Build history of the part. All positions in model axes, mm. A direction names the side the tool comes from. Give positions to 0.01 mm unless a question says otherwise; leave off trailing zeros. Order: outer loops, then holes, each group sorted by start corner. A loop starts at its lowest first (then second) coordinate and runs counter-clockwise, first axis right, second up. Notation, with made-up numbers: (58.25, 11.25) - (111.25, 11.25) arc R17 cw to (111.25, 30.25) - close; hole circle Ø9 at (74, 55). An arc over 180 degrees is marked (long way). Write each question's results on one line, items separated by ' | '. Start each with the question number.
1) Drill centre lines: line 1 along Y through (x, z) = (-4.5, 14); line 2 along Z through (x, y) = (0, 87.5); line 3 along X through (y, z) = (70.5, 50). Where is each one in solid material? Low to high. Write a range as from..to.
2) Drop flat-ended pins along their axis: pin 1 Ø2 at (x, z) = (-12.5, -1) entering from +Y; pin 2 Ø15.5 at (x, z) = (-1.5, 39) entering from +Y; pin 3 Ø3 at (x, y) = (15, 98) entering from +Z; pin 4 Ø6 at (x, z) = (3, -36.5) entering from +Y. Give the stop position or say it passes through.
3) Cut at C-C on y = 81. List the corners of the cut face in (x, z), plus the area to 3 significant figures.
4) Tool access for faces 1 (the face through (13, 100, 44)), 2 (the face through (-4, 5.68, 4)), 3 (the face through (-0.66, 21.367, 14.985)): list every direction of +Z, -Z, +X, -X, +Y, -Y with a clear straight run to the whole face (end or side of a thin tool).
5) Two-plate mould, pull along Y, no slides. Class faces 4 (the face through (0.252, 13.804, -36.289)), 5 (the face through (0.252, 69.587, -44.867)), 6 (the face through (0, 63, 19)), 7 (the face through (-13, 100, 44)): +Y half, -Y half, draft (parallel to the pull), parting line (faces both ways), or undercut.
6) Cut at D-D on x = -2. State how many separate pieces and enclosed holes the cut face has, plus the area to 3 significant figures.
7) Cut at A-A on y = 41. List the corners of the cut face in (x, z).
8) Cut at B-B on z = 47. List the corners of the cut face in (x, y).
from build123d import *

# Parameters (mm, degrees)
SKETCH3_W                               = 40
SKETCH3_H                               = 12
BOSS_EXTRUDE1_DEPTH                     = 12
SKETCH5_R                               = 20
BOSS_EXTRUDE2_DEPTH                     = 20
BOSS_EXTRUDE2_DIRECTION_2_REACH         = 94.331
SKETCH7_R                               = 11.5
BOSS_EXTRUDE4_DEPTH                     = 31
SKETCH8_R                               = 15
BOSS_EXTRUDE5_DEPTH                     = 19
SKETCH9_R                               = 9
CUT_EXTRUDE1_DEPTH                      = 32
BOSS_EXTRUDE6_START                     = 10
BOSS_EXTRUDE6_DEPTH                     = 10
CBORE_FOR_M8_HEX_HEAD_BOLT1_D           = 10
CBORE_FOR_M8_HEX_HEAD_BOLT1_DEPTH       = 43
CBORE_FOR_M8_HEX_HEAD_BOLT1_CBORE_D     = 18.01
CBORE_FOR_M8_HEX_HEAD_BOLT1_CBORE_DEPTH = 5.68
CBORE_FOR_M8_HEX_HEAD_BOLT1_TIP         = 3.004303095
FILLET2_R                               = 18
FILLET3_R                               = 2
FILLET4_R                               = 6
FILLET5_R                               = 2


with BuildPart() as part:
    # Sweep1: sweep along a path in Sketch2
    with BuildLine(Plane(origin=(0, 0, 0), x_dir=(0, 0, -1), z_dir=(1, 0, 0))) as sweep1_path:
        Line((0, 0), (50, 0))
        Line((50, 0), (50, 75))
        Line((50, 75), (-50, 75))
    # Sketch3 → Sweep1 (sweep)
    with BuildSketch(Plane.XY):
        with Locations((0, 6)):
            Rectangle(SKETCH3_W, SKETCH3_H)
    sweep(path=sweep1_path.line, transition=Transition.RIGHT)

    # Sketch4 → Boss-Extrude1 (add)
    with BuildSketch(Plane(origin=(0, 12, 0), x_dir=(1, 0, 0), z_dir=(0, 1, 0))):
        with BuildLine():
            Line((-20, 0), (20, 0))
            ThreePointArc((20, 0), (0, -20), (-20, 0))
        make_face()
    extrude(amount=-BOSS_EXTRUDE1_DEPTH)

    # Sketch5 → Boss-Extrude2 (add)
    with BuildSketch(Plane(origin=(0, 75, 0), x_dir=(1, 0, 0), z_dir=(0, 1, 0))):
        with Locations(Location((0, -50, 0), (0, 0, 270))):
            Circle(SKETCH5_R)
    extrude(amount=BOSS_EXTRUDE2_DEPTH)

    # Boss-Extrude2 direction 2: up to this face of the body (flat: up to its plane)
    boss_extrude2_direction_2_end = Plane(part.part.faces().sort_by_distance((0, 63, 6))[0])
    # Sketch5 → Boss-Extrude2 direction 2 (add, up to the picked face)
    with BuildSketch(Plane(origin=(0, 75, 0), x_dir=(1, 0, 0), z_dir=(0, 1, 0)), mode=Mode.PRIVATE) as boss_extrude2_direction_2_sk1:
        with Locations(Location((0, -50, 0), (0, 0, 270))):
            Circle(SKETCH5_R)
    boss_extrude2_direction_2_tool1 = split(extrude(boss_extrude2_direction_2_sk1.sketch, amount=-BOSS_EXTRUDE2_DIRECTION_2_REACH, mode=Mode.PRIVATE), bisect_by=boss_extrude2_direction_2_end, keep=Keep.BOTH, mode=Mode.PRIVATE)
    add(boss_extrude2_direction_2_tool1.solids().sort_by(Axis((0, 75, 50), (0, -1, 0)))[0])

    # Sketch7 → Boss-Extrude4 (add)
    with BuildSketch(Plane(origin=(0, 12, 0), x_dir=(1, 0, 0), z_dir=(0, 1, 0))):
        with Locations(Location((0, 0, 0), (0, 0, 90))):
            Circle(SKETCH7_R)
    extrude(amount=BOSS_EXTRUDE4_DEPTH)

    # Sketch8 → Boss-Extrude5 (add)
    with BuildSketch(Plane(origin=(0, 12, 0), x_dir=(1, 0, 0), z_dir=(0, 1, 0))):
        with Locations(Location((0, 0, 0), (0, 0, 90))):
            Circle(SKETCH8_R)
    extrude(amount=BOSS_EXTRUDE5_DEPTH)

    # Sketch9 → Cut-Extrude1 (cut)
    with BuildSketch(Plane(origin=(0, 95, 0), x_dir=(1, 0, 0), z_dir=(0, 1, 0))):
        with Locations(Location((0, -50, 0), (0, 0, 270))):
            Circle(SKETCH9_R)
    extrude(amount=-CUT_EXTRUDE1_DEPTH, mode=Mode.SUBTRACT)

    # Sketch10 → Boss-Extrude6 (add)
    with BuildSketch(Plane(origin=(0, 95, 0), x_dir=(1, 0, 0), z_dir=(0, 1, 0)).offset(BOSS_EXTRUDE6_START)):
        with BuildLine():
            Line((-19.078784028, -44), (-6.708203932, -44))
            ThreePointArc((-6.708203932, -44), (-9, -50), (-6.708203932, -56))
            Line((-6.708203932, -56), (-19.078784028, -56))
            ThreePointArc((-19.078784028, -56), (-20, -50), (-19.078784028, -44))
        make_face()
        with BuildLine():
            Line((6.708203932, -44), (19.078784028, -44))
            ThreePointArc((19.078784028, -44), (20, -50), (19.078784028, -56))
            Line((19.078784028, -56), (6.708203932, -56))
            ThreePointArc((6.708203932, -56), (9, -50), (6.708203932, -44))
        make_face()
    extrude(amount=-BOSS_EXTRUDE6_DEPTH)

    # CBORE for M8 Hex Head Bolt1
    with Locations(Plane(origin=(0, 0, 0), x_dir=(-1, 0, 0), z_dir=(0, -1, 0))):
        with Locations((0, 0)):
            CounterBoreHole(CBORE_FOR_M8_HEX_HEAD_BOLT1_D / 2, CBORE_FOR_M8_HEX_HEAD_BOLT1_CBORE_D / 2, CBORE_FOR_M8_HEX_HEAD_BOLT1_CBORE_DEPTH, depth=CBORE_FOR_M8_HEX_HEAD_BOLT1_DEPTH)
            with Locations((0, 0, -(CBORE_FOR_M8_HEX_HEAD_BOLT1_DEPTH + CBORE_FOR_M8_HEX_HEAD_BOLT1_TIP / 2))):  # 118° drill point
                Cone(0, CBORE_FOR_M8_HEX_HEAD_BOLT1_D / 2, CBORE_FOR_M8_HEX_HEAD_BOLT1_TIP, mode=Mode.SUBTRACT)

    # Fillet2
    fillet2_edges = [part.edges().sort_by_distance(p)[0] for p in [
        (0, 75, -50),
        (0, 0, -50),
    ]]
    fillet(fillet2_edges, radius=FILLET2_R)

    # Fillet3
    # the kernel refuses this fillet: 2 mm, written as the material it takes off along each edge
    with BuildSketch(Plane(origin=(20, 18, -32), x_dir=(0, -1, 0), z_dir=(0, 0, 1))) as fillet3_piece_1:
        with BuildLine():
            CenterArc((18 - FILLET3_R, -FILLET3_R), FILLET3_R, 0, 90)
            Line((18 - FILLET3_R, 0), (18, 0))
            Line((18, 0), (18, -FILLET3_R))
        make_face()
    revolve(axis=Axis((20, 18, -32), (1, 0, 0)), revolution_arc=90, mode=Mode.SUBTRACT)
    with BuildSketch(Plane(origin=(20, 18, -50), x_dir=(0, 0, 1), z_dir=(0, 1, 0))) as fillet3_piece_2:
        with BuildLine():
            CenterArc((FILLET3_R, -FILLET3_R), FILLET3_R, 90, 90)
            Line((0, -FILLET3_R), (0, 0))
            Line((0, 0), (FILLET3_R, 0))
        make_face()
    extrude(amount=39, mode=Mode.SUBTRACT)
    with BuildSketch(Plane(origin=(20, 57, -32), x_dir=(0, 0, -1), z_dir=(0, -1, 0))) as fillet3_piece_3:
        with BuildLine():
            CenterArc((18 - FILLET3_R, -FILLET3_R), FILLET3_R, 360, 90)
            Line((18, -FILLET3_R), (18, 0))
            Line((18, 0), (18 - FILLET3_R, 0))
        make_face()
    revolve(axis=Axis((20, 57, -32), (1, 0, 0)), revolution_arc=90, mode=Mode.SUBTRACT)
    with BuildSketch(Plane(origin=(-20, 18, -50), x_dir=(0, 0, 1), z_dir=(0, 1, 0))) as fillet3_piece_4:
        with BuildLine():
            CenterArc((FILLET3_R, FILLET3_R), FILLET3_R, 180, 90)
            Line((0, FILLET3_R), (0, 0))
            Line((0, 0), (FILLET3_R, 0))
        make_face()
    extrude(amount=39, mode=Mode.SUBTRACT)
    with BuildSketch(Plane(origin=(-20, 57, -32), x_dir=(0, 0, -1), z_dir=(0, -1, 0))) as fillet3_piece_5:
        with BuildLine():
            CenterArc((18 - FILLET3_R, FILLET3_R), FILLET3_R, 270, 90)
            Line((18, FILLET3_R), (18, 0))
            Line((18, 0), (18 - FILLET3_R, 0))
        make_face()
    revolve(axis=Axis((-20, 57, -32), (1, 0, 0)), revolution_arc=90, mode=Mode.SUBTRACT)
    with BuildSketch(Plane(origin=(-20, 18, -32), x_dir=(0, -1, 0), z_dir=(0, 0, 1))) as fillet3_piece_6:
        with BuildLine():
            CenterArc((18 - FILLET3_R, FILLET3_R), FILLET3_R, 270, 90)
            Line((18, FILLET3_R), (18, 0))
            Line((18, 0), (18 - FILLET3_R, 0))
        make_face()
    revolve(axis=Axis((-20, 18, -32), (1, 0, 0)), revolution_arc=90, mode=Mode.SUBTRACT)
    with BuildSketch(Plane(origin=(20, 75, -32), x_dir=(0, -1, 0), z_dir=(0, 0, 1))) as fillet3_piece_7_section:
        with BuildLine():
            CenterArc((FILLET3_R, -FILLET3_R), FILLET3_R, 90, 90)
            Line((0, -FILLET3_R), (0, 0))
            Line((0, 0), (FILLET3_R, 0))
        make_face()
    fillet3_piece_7 = extrude(amount=87, mode=Mode.PRIVATE)
    fillet3_piece_7 = fillet3_piece_7 - Plane(origin=(0, 74.534164158, 50), x_dir=(0, 0, 1), z_dir=(0, -1, 0)) * Cylinder(20, 183, mode=Mode.PRIVATE)
    add(fillet3_piece_7, mode=Mode.SUBTRACT)
    with BuildSketch(Plane(origin=(-20, 75, -32), x_dir=(0, -1, 0), z_dir=(0, 0, 1))) as fillet3_piece_8_section:
        with BuildLine():
            CenterArc((FILLET3_R, FILLET3_R), FILLET3_R, 180, 90)
            Line((0, FILLET3_R), (0, 0))
            Line((0, 0), (FILLET3_R, 0))
        make_face()
    fillet3_piece_8 = extrude(amount=87, mode=Mode.PRIVATE)
    fillet3_piece_8 = fillet3_piece_8 - Plane(origin=(0, 74.534164167, 50), x_dir=(0, 0, 1), z_dir=(0, -1, 0)) * Cylinder(20, 183, mode=Mode.PRIVATE)
    add(fillet3_piece_8, mode=Mode.SUBTRACT)
    with BuildSketch(Plane(origin=(-20, 0, 0), x_dir=(1, 0, 0), z_dir=(0, 0, -1))) as fillet3_piece_9:
        with BuildLine():
            CenterArc((FILLET3_R, -FILLET3_R), FILLET3_R, 90, 90)
            Line((0, -FILLET3_R), (0, 0))
            Line((0, 0), (FILLET3_R, 0))
        make_face()
    extrude(amount=32, mode=Mode.SUBTRACT)
    with BuildSketch(Plane(origin=(0, 0, 0), x_dir=(1, 0, 0), z_dir=(0, 0, -1))) as fillet3_piece_10:
        with BuildLine():
            CenterArc((20 - FILLET3_R, -FILLET3_R), FILLET3_R, 0, 90)
            Line((20, -FILLET3_R), (20, 0))
            Line((20, 0), (20 - FILLET3_R, 0))
        make_face()
    revolve(axis=Axis((0, 0, 0), (0, -1, 0)), revolution_arc=180, mode=Mode.SUBTRACT)
    with BuildSketch(Plane(origin=(20, 0, 0), x_dir=(-1, 0, 0), z_dir=(0, 0, -1))) as fillet3_piece_11:
        with BuildLine():
            CenterArc((FILLET3_R, FILLET3_R), FILLET3_R, 180, 90)
            Line((0, FILLET3_R), (0, 0))
            Line((0, 0), (FILLET3_R, 0))
        make_face()
    extrude(amount=32, mode=Mode.SUBTRACT)

    # Fillet4
    fillet4_edges = [part.edges().sort_by_distance(p)[0] for p in [
        (0, 63, -38),
        (0, 12, -38),
    ]]
    fillet(fillet4_edges, radius=FILLET4_R)

    # Fillet5
    fillet5_edges = [part.edges().sort_by_distance(p)[0] for p in [
        (20, 63, 9),
        (-20, 63, 9),
        (-20, 37.5, -38),
        (20, 37.5, -38),
        (20, 61.242640687, -36.242640687),
        (20, 61.242640687, -36.242640687),
        (-20, 61.242640687, -36.242640687),
        (-20, 61.242640687, -36.242640687),
        (20, 13.757359313, -36.242640687),
        (20, 13.757359313, -36.242640687),
        (-20, 13.757359313, -36.242640687),
        (-20, 13.757359313, -36.242640687),
        (-20, 12, -16),
        (0, 12, 20),
        (20, 12, -16),
        (-14.142135624, 63, 64.142135624),
    ]]
    fillet(fillet5_edges, radius=FILLET5_R)


solid = part.part
Results:
1) line 1: 0..31, 63..75 | line 2: 30..41, 59..70 | line 3: -20..-9, 9..20
2) pin 1: y = 75 | pin 2: y = 105 | pin 3: z = 56 | pin 4: y = 74.94
3) outline: circle Ø40 at (0, 50); hole circle Ø18 at (0, 50) | area: 1,000 mm^2
4) face 1: -Z, +X, -X, +Y | face 2: -Y | face 3: none
5) face 4: undercut | face 5: +Y half | face 6: undercut | face 7: draft
6) separate pieces: 3 | enclosed holes: 0 | area: 3,390 mm^2
7) outline: (-20, -48) arc R2 ccw to (-18, -50) - (18, -50) arc R2 ccw to (20, -48) - (20, -40) arc R2 ccw to (18, -38) - (-18, -38) arc R2 ccw to (-20, -40) - close; circle Ø23 at (0, 0); hole circle Ø10 at (0, 0)
8) outline: (-20, 65) arc R2 ccw to (-18, 63) - (-8.49, 63) - (-8.49, 105) - (-19.77, 105) - (-19.77, 73.92) arc R2 ccw to (-20, 73) - close; (8.49, 63) - (18, 63) arc R2 ccw to (20, 65) - (20, 73) arc R2 ccw to (19.77, 73.92) - (19.77, 105) - (8.49, 105) - close
